Check sheet for the modelled part. Datum: model origin and axes. Units: mm. Face numbers are marked on the shaded views. A direction names the side the tool comes from. Give positions to 0.01 mm unless a question says otherwise; leave off trailing zeros. Write each loop counter-clockwise with the first axis right and the second up, starting at its lowest first coordinate (ties: lowest second). Pieces come first, ordered by that corner, then holes. Notation, with made-up numbers: (-35, -13) -> (-23, -13) arc R24 ccw to (-23, 23) -> close; hole circle Ø6 at (36.5, 68.25). An arc over 180 degrees is marked (long way). Use a Markdown table: item, result. Add a question column.
1. Cross-section at C-C (x = 101). Enter the section's corners in (y, z) (3 decimals).
2. Cross-section at A-A (z = 6). Enter the section's corners in (x, y) (3 decimals).
3. Cross-section at B-B (y = -29). Enter the section's corners in (x, z) (3 decimals), then the cut area to 3 significant figures.
4. Gauge pin test, flat ends, axial feed: P1, Ø10, axis at x = -24, y = -11.5, coming from the +Z side; P2, Ø5, axis at y = -11, z = 57, coming from the -X side; P3, Ø4, axis at x = 42, y = -48, coming from the -Z side (3 decimals); P4, Ø18.5, axis at y = 3.5, z = 6, coming from the +X side (3 decimals). Record the tip position at first contact, or that the pin passes through.
5. Scan lines: probe 1 along Y at (x, z) = (32, 49); probe 2 along Z at (x, y) = (18, -55) (3 decimals); probe 3 along X at (y, z) = (31.5, 6) (3 decimals). Record each from-to range of solid material in increasing order. Write a range as [from, to].
6. Set-up check for the marked faces 1, 2 and 3: record each of +Z, -Z, +X, -X, +Y, -Y from which the full face is reachable in a straight line by a thin tool's end or side.
from build123d import *

# Parameters (mm, degrees)
F1_DEPTH = 63.5
F2_DEPTH = 7.9375
F0_W     = 25.4
F0_H     = 19.05
F3_DEPTH = 25.4
F5_R     = 6.35


with BuildPart() as f1:
    # F0 (on Front) → F1 (new body, symmetric)
    with BuildSketch(Plane.XZ):
        Polygon((41.275, -9.525), (41.275, 9.525), (22.225, 9.525), (-41.275, 9.525), (-41.275, -9.525), align=None)
    extrude(amount=F1_DEPTH, both=True)

    # F0 (on Front) → F2 (join, symmetric)
    with BuildSketch(Plane.XZ):
        with BuildLine():
            Line((-41.275, 9.525), (22.225, 9.525))
            Line((22.225, 9.525), (22.225, 27.0002))
            ThreePointArc((22.225, 27.0002), (31.6817510104, 50.8983990619), (54.9307362006, 61.8546185605))
            add(Edge.make_bspline(
                [(-41.275, 9.525), (-41.7675076432, 41.9812705622), (6.5603954345, 60.0669286801), (54.9307362006, 61.8546185605)],
                knots=[0, 0, 0, 0, 109.8248144815, 109.8248144815, 109.8248144815, 109.8248144815], degree=3))
        make_face()
    extrude(amount=F2_DEPTH, both=True)

    # F0 (on Front) → F3 (join, symmetric)
    with BuildSketch(Plane.XZ):
        with BuildLine():
            Line((22.225, 9.525), (41.275, 9.525))
            Line((41.275, 9.525), (41.275, 27.0002))
            ThreePointArc((41.275, 27.0002), (45.9246798487, 38.2255201513), (57.15, 42.8752))
            Line((57.15, 42.8752), (60.325, 42.8752))
            Line((60.325, 42.8752), (60.325, 61.9252))
            Line((60.325, 61.9252), (57.15, 61.9252))
            add(Edge.make_bspline(
                [(54.9307362006, 61.8546185605), (55.6705390451, 61.8819604819), (56.4103518168, 61.905489927), (57.15, 61.9252)],
                knots=[109.8248144815, 109.8248144815, 109.8248144815, 109.8248144815, 111.5045361635, 111.5045361635, 111.5045361635, 111.5045361635], degree=3))
            ThreePointArc((54.9307362006, 61.8546185605), (31.6817510104, 50.8983990619), (22.225, 27.0002))
            Line((22.225, 27.0002), (22.225, 9.525))
        make_face()
        with Locations((73.025, 52.4002)):
            Rectangle(F0_W, F0_H)
    extrude(amount=F3_DEPTH, both=True)

    # F0 (on Front) → F4 (revolve)
    with BuildSketch(Plane.XZ):
        Polygon((85.725, 61.9252), (85.725, 42.8752), (85.725, 38.1), (111.125, 38.1), (111.125, 66.675), (85.725, 66.675), align=None)
    revolve(axis=Axis((85.725, 0, 52.3875), (0, 0, 1)))

    # F5
    f5_edges = [f1.edges().sort_by_distance(p)[0] for p in [
        (41.275, -63.5, 0),
        (-41.275, -63.5, 0),
        (-41.275, 63.5, 0),
        (41.275, 63.5, 0),
    ]]
    fillet(f5_edges, radius=F5_R)


solid = f1.part
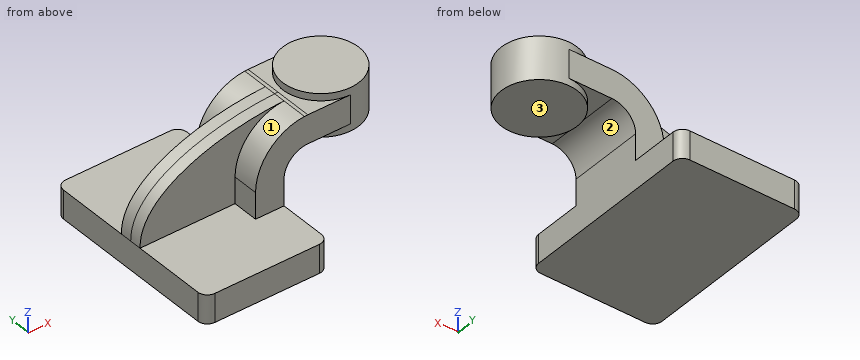
Worked answers:
| question | item | result |
|---|---|---|
| 1 | outline | (-20.294, 38.1) -> (20.294, 38.1) -> (20.294, 66.675) -> (-20.294, 66.675) -> close |
| 2 | outline | (-41.275, -57.15) arc R6.35 ccw to (-34.925, -63.5) -> (34.925, -63.5) arc R6.35 ccw to (41.275, -57.15) -> (41.275, 57.15) arc R6.35 ccw to (34.925, 63.5) -> (-34.925, 63.5) arc R6.35 ccw to (-41.275, 57.15) -> close |
| 3 | outline | (-41.275, -9.525) -> (41.275, -9.525) -> (41.275, 9.525) -> (-41.275, 9.525) -> close |
| 3 | area | 1,570 mm² |
| 4 | P1 | stops at z = 42.15 |
| 4 | P2 | stops at x = 35.62 |
| 4 | P3 | stops at z = -9.525 |
| 4 | P4 | stops at x = 41.275 |
| 5 | probe 1 | y = [-25.4, 25.4] |
| 5 | probe 2 | z = [-9.525, 9.525] |
| 5 | probe 3 | x = [-41.275, 41.275] |
| 6 | face 1 | +Z, -X, -Y |
| 6 | face 2 | -Z, +Y, -Y |
| 6 | face 3 | -Z, +X, +Y, -Y |
